Design review of the part built by this model. Coordinates are the model's own, in mm. A direction names the side the tool comes from. Coordinates: 2 decimals unless noted, no trailing zeros. Write each loop counter-clockwise with the first axis right and the second up, starting at its lowest first coordinate (ties: lowest second). Pieces come first, ordered by that corner, then holes. Notation, with made-up numbers: M -31,59 L 15,59 A29 cw 15,84 Z; hole C 16.25,20 d1. An arc over 180 degrees is marked long. Write each question's results on one line, items separated by ' | '. Start each with the question number.
```python
from build123d import *

# Parameters (mm, degrees)
BOSS_EXTRUDE1_DEPTH       = 3
BOSS_EXTRUDE2_DEPTH       = 20
CHAMFER1_SIZE             = 20
SKETCH9_R                 = 1.75
CUT_EXTRUDE6_DEPTH        = 192.426225998
CHAMFER2_SIZE             = 10
CHAMFER2_SIZE2            = 7.002075382
SKETCH12_W                = 40
SKETCH12_H                = 120
BOSS_EXTRUDE3_DEPTH       = 30
CUT_EXTRUDE8_DEPTH        = 120
CUT_EXTRUDE9_DEPTH        = 194.217494032
FILLET2_R                 = 20
SKETCH16_R                = 1.75
CUT_EXTRUDE10_DEPTH       = 193.727787374
LPATTERN1_COUNT           = 7
LPATTERN1_PITCH           = 10
SKETCH17_R                = 1.75
CUT_EXTRUDE11_DEPTH       = 193.727787374
LPATTERN2_COUNT           = 2
LPATTERN2_PITCH           = 12.5
MIRROR4_COPY_1_SKETCH_R   = 1.75
MIRROR4_COPY_1_DEPTH      = 193.727787374
SKETCH18_R                = 1.75
CUT_EXTRUDE12_DEPTH       = 193.727787374
LPATTERN3_COUNT           = 10
LPATTERN3_PITCH           = 10
LPATTERN4_COUNT           = 2
LPATTERN4_PITCH           = 12.5
LPATTERN4_COPY_1_SKETCH_R = 1.75
LPATTERN4_COPY_1_DEPTH    = 193.727787374
LPATTERN4_COPY_2_SKETCH_R = 1.75
LPATTERN4_COPY_2_DEPTH    = 193.727787374
LPATTERN4_COPY_3_SKETCH_R = 1.75
LPATTERN4_COPY_3_DEPTH    = 193.727787374
LPATTERN4_COPY_4_SKETCH_R = 1.75
LPATTERN4_COPY_4_DEPTH    = 193.727787374
LPATTERN4_COPY_5_SKETCH_R = 1.75
LPATTERN4_COPY_5_DEPTH    = 193.727787374
LPATTERN4_COPY_6_SKETCH_R = 1.75
LPATTERN4_COPY_6_DEPTH    = 193.727787374
LPATTERN4_COPY_7_SKETCH_R = 1.75
LPATTERN4_COPY_7_DEPTH    = 193.727787374
LPATTERN4_COPY_8_SKETCH_R = 1.75
LPATTERN4_COPY_8_DEPTH    = 193.727787374
LPATTERN4_COPY_9_SKETCH_R = 1.75
LPATTERN4_COPY_9_DEPTH    = 193.727787374


with BuildPart() as part:
    # Sketch1 → Boss-Extrude1 (new body)
    with BuildSketch(Plane(origin=(0, 0, 0), x_dir=(1, 0, 0), z_dir=(0, 1, 0))):
        Polygon((100, 60), (100, -60), (70, -60), (70, -128), (-70, -128), (-70, -60), (-100, -60), (-100, 60), (-27.5, 60), (-27.5, 140), (-100, 140), (-100, 142), (-70, 162), (70, 162), (100, 142), (100, 140), (27.5, 140), (27.5, 60), align=None)
    extrude(amount=BOSS_EXTRUDE1_DEPTH)

    # Sketch8 → Boss-Extrude2 (add)
    with BuildSketch(Plane(origin=(0, 3, 0), x_dir=(1, 0, 0), z_dir=(0, 1, 0))):
        Polygon((-100, 140), (100, 140), (100, 142), (70, 162), (-70, 162), (-100, 142), align=None)
    extrude(amount=BOSS_EXTRUDE2_DEPTH)

    # Chamfer1
    # the kernel refuses this chamfer: 20 mm, written as the material it takes off along each edge
    with BuildSketch(Plane(origin=(121.433659759, 23, -162), x_dir=(0, -0.9996219169112968, -0.027495876610586317), z_dir=(-1, 0, 0))) as chamfer1_piece_1:
        Polygon((CHAMFER1_SIZE * 0.999621916911, CHAMFER1_SIZE * 0.0274958766106), (-CHAMFER1_SIZE * 0.0274958766106, CHAMFER1_SIZE * 0.999621916911), (0, 0), align=None)
    extrude(amount=242.867319519, mode=Mode.SUBTRACT)
    with BuildSketch(Plane(origin=(-100, 23, -193.433659759), x_dir=(-0.027495876610586317, -0.9996219169112968, 0), z_dir=(0, 0, 1))) as chamfer1_piece_2:
        Polygon((CHAMFER1_SIZE * 0.999621916911, CHAMFER1_SIZE * 0.0274958766106), (-CHAMFER1_SIZE * 0.0274958766106, CHAMFER1_SIZE * 0.999621916911), (0, 0), align=None)
    extrude(amount=104.867319519, mode=Mode.SUBTRACT)
    with BuildSketch(Plane(origin=(100, 23, -88.566340241), x_dir=(-0.9996219169112968, 0.027495876610586317, 0), z_dir=(0, 0, -1))) as chamfer1_piece_3:
        Polygon((CHAMFER1_SIZE * 0.999621916911, -CHAMFER1_SIZE * 0.0274958766106), (-CHAMFER1_SIZE * 0.0274958766106, -CHAMFER1_SIZE * 0.999621916911), (0, 0), align=None)
    extrude(amount=104.867319519, mode=Mode.SUBTRACT)

    # Sketch9 → Cut-Extrude6 (cut, through all)
    with BuildSketch(Plane(origin=(0, 3, 0), x_dir=(1, 0, 0), z_dir=(0, 1, 0))):
        with Locations(Location((-15, 100, 0), (0, 0, 270))):
            Circle(SKETCH9_R)
        with Locations(Location((15, 100, 0), (0, 0, 270))):
            Circle(SKETCH9_R)
        with Locations(Location((0, 115, 0), (0, 0, 270))):
            Circle(SKETCH9_R)
        with Locations(Location((0, 85, 0), (0, 0, 270))):
            Circle(SKETCH9_R)
    extrude(amount=-CUT_EXTRUDE6_DEPTH, mode=Mode.SUBTRACT)

    # Chamfer2
    chamfer2_edges = [part.edges().sort_by_distance(p)[0] for p in [
        (0, 3, -140),
    ]]
    chamfer2_side = [part.faces().sort_by_distance(p)[0] for p in [
        (0, 11.429781082, -140),
    ]]
    chamfer(chamfer2_edges, length=CHAMFER2_SIZE, length2=CHAMFER2_SIZE2, reference=chamfer2_side[0])

    # Sketch12 → Boss-Extrude3 (add)
    with BuildSketch(Plane(origin=(0, 3, 0), x_dir=(1, 0, 0), z_dir=(0, 1, 0))):
        with Locations((-80, 0)):
            Rectangle(SKETCH12_W, SKETCH12_H)
    boss_extrude3 = extrude(amount=BOSS_EXTRUDE3_DEPTH)

    # Sketch13 → Cut-Extrude8 (cut)
    with BuildSketch(Plane.XY.offset(60)):
        with BuildLine():
            Line((-97, 33), (-60, 33))
            Line((-60, 33), (-60, 3))
            ThreePointArc((-60, 3), (-83.63033668, 11.672584761), (-97, 33))
        make_face()
    cut_extrude8 = extrude(amount=-CUT_EXTRUDE8_DEPTH, mode=Mode.SUBTRACT)

    # Sketch14 → Cut-Extrude9 (cut, through all)
    with BuildSketch(Plane.XZ):
        with BuildLine():
            Line((-31.303743975, -60), (-94.382349042, -60))
            ThreePointArc((-94.382349042, -60), (-62.843046509, -39.350555542), (-31.303743975, -60))
        make_face()
    cut_extrude9 = extrude(amount=-CUT_EXTRUDE9_DEPTH, mode=Mode.SUBTRACT)

    # Mirror3: Boss-Extrude3, Cut-Extrude8, Cut-Extrude9 across plane
    add(boss_extrude3.mirror(Plane(origin=(0, 0, 0), x_dir=(0, 0, 1), z_dir=(1, 0, 0))))
    add(cut_extrude8.mirror(Plane(origin=(0, 0, 0), x_dir=(0, 0, 1), z_dir=(1, 0, 0))), mode=Mode.SUBTRACT)
    add(cut_extrude9.mirror(Plane(origin=(0, 0, 0), x_dir=(0, 0, 1), z_dir=(1, 0, 0))), mode=Mode.SUBTRACT)

    # Fillet2
    fillet2_edges = [part.edges().sort_by_distance(p)[0] for p in [
        (-100, 0, 0),
        (100, 0, 0),
    ]]
    fillet(fillet2_edges, radius=FILLET2_R)

    # Sketch16 → Cut-Extrude10 (cut, through all)
    with BuildSketch(Plane(origin=(0, 3, 0), x_dir=(1, 0, 0), z_dir=(0, 1, 0))):
        with Locations(Location((-17.25, 49.727630158, 0), (0, 0, 270))):
            Circle(SKETCH16_R)
        with Locations(Location((17.25, 49.727630158, 0), (0, 0, 270))):
            Circle(SKETCH16_R)
    cut_extrude10 = extrude(amount=-CUT_EXTRUDE10_DEPTH, mode=Mode.SUBTRACT)

    # LPattern1: Cut-Extrude10 ×7
    with Locations(*[(0, 0, i * LPATTERN1_PITCH) for i in range(1, LPATTERN1_COUNT)]):
        add(cut_extrude10, mode=Mode.SUBTRACT)

    # Sketch17 → Cut-Extrude11 (cut, through all)
    with BuildSketch(Plane(origin=(0, 3, 0), x_dir=(1, 0, 0), z_dir=(0, 1, 0))):
        with Locations(Location((-60, -118, 0), (0, 0, 270))):
            Circle(SKETCH17_R)
        with Locations(Location((-60, -93, 0), (0, 0, 270))):
            Circle(SKETCH17_R)
    cut_extrude11 = extrude(amount=-CUT_EXTRUDE11_DEPTH, mode=Mode.SUBTRACT)

    # LPattern2: Cut-Extrude11 ×2
    with Locations(*[(0, 0, -i * LPATTERN2_PITCH) for i in range(1, LPATTERN2_COUNT)]):
        add(cut_extrude11, mode=Mode.SUBTRACT)

    # Mirror4: Cut-Extrude11 across plane
    add(cut_extrude11.mirror(Plane(origin=(0, 0, 0), x_dir=(0, 0, 1), z_dir=(1, 0, 0))), mode=Mode.SUBTRACT)

    # Mirror4 copy 1 sketch → Mirror4 copy 1 (cut, through all)
    with BuildSketch(Plane(origin=(0, 3, -12.5), x_dir=(-1, 0, 0), z_dir=(0, 1, 0))):
        with Locations((-60, 118)):
            Circle(MIRROR4_COPY_1_SKETCH_R)
        with Locations((-60, 93)):
            Circle(MIRROR4_COPY_1_SKETCH_R)
    extrude(amount=-MIRROR4_COPY_1_DEPTH, mode=Mode.SUBTRACT)

    # Sketch18 → Cut-Extrude12 (cut, through all)
    with BuildSketch(Plane(origin=(0, 3, 0), x_dir=(1, 0, 0), z_dir=(0, 1, 0))):
        with Locations(Location((-45, -82, 0), (0, 0, 270))):
            Circle(SKETCH18_R)
        with Locations(Location((-45, -65, 0), (0, 0, 270))):
            Circle(SKETCH18_R)
    cut_extrude12 = extrude(amount=-CUT_EXTRUDE12_DEPTH, mode=Mode.SUBTRACT)

    # LPattern3: Cut-Extrude12 ×10
    with Locations(*[(i * LPATTERN3_PITCH, 0, 0) for i in range(1, LPATTERN3_COUNT)]):
        add(cut_extrude12, mode=Mode.SUBTRACT)

    # LPattern4: Cut-Extrude12 ×2
    with Locations(*[(0, 0, i * LPATTERN4_PITCH) for i in range(1, LPATTERN4_COUNT)]):
        add(cut_extrude12, mode=Mode.SUBTRACT)

    # LPattern4 copy 1 sketch → LPattern4 copy 1 (cut, through all)
    with BuildSketch(Plane(origin=(10, 3, 12.5), x_dir=(1, 0, 0), z_dir=(0, 1, 0))):
        with Locations(Location((-45, -82, 0), (0, 0, 270))):
            Circle(LPATTERN4_COPY_1_SKETCH_R)
        with Locations(Location((-45, -65, 0), (0, 0, 270))):
            Circle(LPATTERN4_COPY_1_SKETCH_R)
    extrude(amount=-LPATTERN4_COPY_1_DEPTH, mode=Mode.SUBTRACT)

    # LPattern4 copy 2 sketch → LPattern4 copy 2 (cut, through all)
    with BuildSketch(Plane(origin=(20, 3, 12.5), x_dir=(1, 0, 0), z_dir=(0, 1, 0))):
        with Locations(Location((-45, -82, 0), (0, 0, 270))):
            Circle(LPATTERN4_COPY_2_SKETCH_R)
        with Locations(Location((-45, -65, 0), (0, 0, 270))):
            Circle(LPATTERN4_COPY_2_SKETCH_R)
    extrude(amount=-LPATTERN4_COPY_2_DEPTH, mode=Mode.SUBTRACT)

    # LPattern4 copy 3 sketch → LPattern4 copy 3 (cut, through all)
    with BuildSketch(Plane(origin=(30, 3, 12.5), x_dir=(1, 0, 0), z_dir=(0, 1, 0))):
        with Locations(Location((-45, -82, 0), (0, 0, 270))):
            Circle(LPATTERN4_COPY_3_SKETCH_R)
        with Locations(Location((-45, -65, 0), (0, 0, 270))):
            Circle(LPATTERN4_COPY_3_SKETCH_R)
    extrude(amount=-LPATTERN4_COPY_3_DEPTH, mode=Mode.SUBTRACT)

    # LPattern4 copy 4 sketch → LPattern4 copy 4 (cut, through all)
    with BuildSketch(Plane(origin=(40, 3, 12.5), x_dir=(1, 0, 0), z_dir=(0, 1, 0))):
        with Locations(Location((-45, -82, 0), (0, 0, 270))):
            Circle(LPATTERN4_COPY_4_SKETCH_R)
        with Locations(Location((-45, -65, 0), (0, 0, 270))):
            Circle(LPATTERN4_COPY_4_SKETCH_R)
    extrude(amount=-LPATTERN4_COPY_4_DEPTH, mode=Mode.SUBTRACT)

    # LPattern4 copy 5 sketch → LPattern4 copy 5 (cut, through all)
    with BuildSketch(Plane(origin=(50, 3, 12.5), x_dir=(1, 0, 0), z_dir=(0, 1, 0))):
        with Locations(Location((-45, -82, 0), (0, 0, 270))):
            Circle(LPATTERN4_COPY_5_SKETCH_R)
        with Locations(Location((-45, -65, 0), (0, 0, 270))):
            Circle(LPATTERN4_COPY_5_SKETCH_R)
    extrude(amount=-LPATTERN4_COPY_5_DEPTH, mode=Mode.SUBTRACT)

    # LPattern4 copy 6 sketch → LPattern4 copy 6 (cut, through all)
    with BuildSketch(Plane(origin=(60, 3, 12.5), x_dir=(1, 0, 0), z_dir=(0, 1, 0))):
        with Locations(Location((-45, -82, 0), (0, 0, 270))):
            Circle(LPATTERN4_COPY_6_SKETCH_R)
        with Locations(Location((-45, -65, 0), (0, 0, 270))):
            Circle(LPATTERN4_COPY_6_SKETCH_R)
    extrude(amount=-LPATTERN4_COPY_6_DEPTH, mode=Mode.SUBTRACT)

    # LPattern4 copy 7 sketch → LPattern4 copy 7 (cut, through all)
    with BuildSketch(Plane(origin=(70, 3, 12.5), x_dir=(1, 0, 0), z_dir=(0, 1, 0))):
        with Locations(Location((-45, -82, 0), (0, 0, 270))):
            Circle(LPATTERN4_COPY_7_SKETCH_R)
        with Locations(Location((-45, -65, 0), (0, 0, 270))):
            Circle(LPATTERN4_COPY_7_SKETCH_R)
    extrude(amount=-LPATTERN4_COPY_7_DEPTH, mode=Mode.SUBTRACT)

    # LPattern4 copy 8 sketch → LPattern4 copy 8 (cut, through all)
    with BuildSketch(Plane(origin=(80, 3, 12.5), x_dir=(1, 0, 0), z_dir=(0, 1, 0))):
        with Locations(Location((-45, -82, 0), (0, 0, 270))):
            Circle(LPATTERN4_COPY_8_SKETCH_R)
        with Locations(Location((-45, -65, 0), (0, 0, 270))):
            Circle(LPATTERN4_COPY_8_SKETCH_R)
    extrude(amount=-LPATTERN4_COPY_8_DEPTH, mode=Mode.SUBTRACT)

    # LPattern4 copy 9 sketch → LPattern4 copy 9 (cut, through all)
    with BuildSketch(Plane(origin=(90, 3, 12.5), x_dir=(1, 0, 0), z_dir=(0, 1, 0))):
        with Locations(Location((-45, -82, 0), (0, 0, 270))):
            Circle(LPATTERN4_COPY_9_SKETCH_R)
        with Locations(Location((-45, -65, 0), (0, 0, 270))):
            Circle(LPATTERN4_COPY_9_SKETCH_R)
    extrude(amount=-LPATTERN4_COPY_9_DEPTH, mode=Mode.SUBTRACT)


solid = part.part
```
Item 1: Draft analysis for pull direction Z (two halves, no side actions). For faces 4 (the flat face through (85, 6, -152)), 5 (the flat face through (-27.5, 2.6, -105.7)), 6 (the flat face through (-100, 26, 1)), 7 (the flat face through (27.5, 2.6, -106.1)), state which applies: released by +Z, released by -Z, zero draft, split by the parting line, or undercut.
Item 2: We need section B-B on z = 45.5. State the section outline as (x, y) points, then the cut area to 3 significant figures.
Item 3: We need section A-A on x = -75.5. State the section outline as (y, z) points, then the cut area to 3 significant figures.
Item 4: We need section C-C on y = 29. State the section outline as (x, z) points, then the cut area to 3 significant figures.
Item 5: For faces 1 (the flat face through (-90, 13, -144)), 2 (the flat face through (1, 3, 25)), 3 (the flat face through (90, 13, -144)), list the 3-axis set-ups (+Z, -Z, +X, -X, +Y, -Y) from which the entire face can be reached by the end or side of a thin tool; tool diameter is ignored.
Item 6: Wall thickness on L1, parallel to X at y = 1.45, z = 105.5; L2, parallel to Z at x = 0.5, y = 2; L3, parallel to Z at x = 61, y = 2.5: over which ranges is each line inside the solid? List them lowest first.
Item 7: We need section D-D on z = -120.5. State the section outline as (x, y) points, then the cut area to 3 significant figures.
Item 8: Insertion check: pin 1 Ø4.5 at (x, z) = (17.25, -39.73) entering from +Y; pin 2 Ø5.5 at (x, z) = (15, 94.5) entering from -Y; pin 3 Ø4.5 at (x, y) = (-98.5, 25.5) entering from -Z; pin 4 Ø3 at (x, y) = (2.5, 9) entering from +Z. Each pin has a flat end and moves straight along its axis. Give the tip position at first contact, or say it passes through.
Answer:
1) face 4: released by -Z | face 5: undercut | face 6: zero draft | face 7: undercut
2) outline: M -100,20 A20 ccw -80,0 L 80,0 A20 ccw 100,20 L 100,33 L 97,33 A38.89 cw 60,3 L -60,3 A38.89 cw -97,33 L -100,33 Z | area: 1,190 mm^2
3) outline: M 0,-158.33 L 6.67,-158.33 L 23,-142 L 23,-140 L 0,-140 Z; M 0,-41.76 L 6.6,-41.76 L 6.6,60 L 0,60 Z | area: 960 mm^2
4) outline: M -100,-60 L -95.83,-60 L -95.83,60 L -100,60 Z; M 95.83,-60 L 100,-60 L 100,60 L 95.83,60 Z | area: 1,000 mm^2
5) face 1: -Z, -X, +Y | face 2: +Z, +Y | face 3: -Z, +X, +Y
6) L1: x = -70 to -61.75, -58.25 to 58.25, 61.75 to 70 | L2: z = -162 to -116.68, -113.32 to -86.68, -83.32 to 128 | L3: z = -162 to -140, -39.4 to 79.06, 81.94 to 91.56, 94.44 to 104.06, 106.94 to 116.56, 119.44 to 128
7) outline: M -27.5,0 L 27.5,0 L 27.5,3 L -27.5,3 Z | area: 165 mm^2
8) pin 1: stops at y = 3 | pin 2: stops at y = 0 | pin 3: stops at z = -60 | pin 4: stops at z = -136.15
